```python
from build123d import *

# Parameters (mm, degrees)
F0_R     = 3
F1_DEPTH = 3.95
F0_R_2   = 2.499
F0_R_3   = 2.495
F2_DEPTH = 3.45
F3_R     = 3.69999


# Not quite as in the source:
# - a fillet or chamfer is up to 0.001 mm smaller than in the source, because OpenCascade refuses the exact size


with BuildPart() as f1:
    # F0 (on Front) → F1 (new body, symmetric)
    with BuildSketch(Plane.XZ):
        Polygon((15.7, -3.7), (15.7, 0), (15.7, 3.7), (-15.7, 3.7), (-15.7, -3.7), align=None)
        with BuildLine():
            ThreePointArc((-12.8998169675, 2.8618751589), (-11.9998409744, 2.9999999958), (-11.0998796299, 2.8617797468))
            Line((-11.0998796299, 2.8617797468), (-11.0998796299, 0.8996879915))
            Line((-11.0998796299, 0.8996879915), (-9.1380842923, 0.8996879915))
            ThreePointArc((-9.1380842923, 0.8996879915), (-9.0000000001, -2.51387e-05), (-9.1380993707, -0.8997359546))
            Line((-9.1380993707, -0.8997359546), (-11.0998796299, -0.8997359546))
            Line((-11.0998796299, -0.8997359546), (-11.0998796299, -2.8617797468))
            ThreePointArc((-11.0998796299, -2.8617797468), (-11.9998409744, -2.9999999958), (-12.8998169675, -2.8618751589))
            Line((-12.8998169675, -2.8618751589), (-12.8998169675, -0.8997359546))
            Line((-12.8998169675, -0.8997359546), (-14.8619006293, -0.8997359546))
            ThreePointArc((-14.8619006293, -0.8997359546), (-14.9999999999, -2.51387e-05), (-14.8619157077, 0.8996879915))
            Line((-14.8619157077, 0.8996879915), (-12.8998169675, 0.8996879915))
            Line((-12.8998169675, 0.8996879915), (-12.8998169675, 2.8618751589))
        make_face(mode=Mode.SUBTRACT)
        with Locations((-4, 0)):
            Circle(F0_R, mode=Mode.SUBTRACT)
        with Locations((4, 0)):
            Circle(F0_R, mode=Mode.SUBTRACT)
        with Locations((12, 0)):
            Circle(F0_R, mode=Mode.SUBTRACT)
    extrude(amount=F1_DEPTH, both=True)

    # F0 (on Front) → F2 (join, symmetric)
    with BuildSketch(Plane.XZ):
        with Locations((-4, 0)):
            Circle(F0_R)
        with Locations((-4, 0)):
            Circle(F0_R_2, mode=Mode.SUBTRACT)
        with Locations((4, 0)):
            Circle(F0_R)
        with Locations((4, 0)):
            Circle(F0_R_3, mode=Mode.SUBTRACT)
        with Locations((12, 0)):
            Circle(F0_R)
        with Locations((12, 0)):
            Circle(F0_R_2, mode=Mode.SUBTRACT)
    extrude(amount=F2_DEPTH, both=True)

    # F3 (radius 3.7 in the source; OpenCascade refuses exactly that, so slightly less here)
    f3_edges = [f1.edges().sort_by_distance(p)[0] for p in [
        (-15.7, 0, 3.7),
        (-15.7, 0, -3.7),
        (15.7, 0, 3.7),
        (15.7, 0, -3.7),
    ]]
    fillet(f3_edges, radius=F3_R)


solid = f1.part
```
Part model, mm, in its own coordinate system. A direction names the side the tool comes from. Round coordinates to 2 decimals unless told otherwise and drop trailing zeros. Write each loop counter-clockwise with the first axis right and the second up, starting at its lowest first coordinate (ties: lowest second). Pieces come first, ordered by that corner, then holes.
Item 1: Probe L1, parallel to Z at x = 4, y = -3.7; L2, parallel to Z at x = 12, y = -1.25; L3, parallel to X at y = 0.5, z = 2.25. List the from-to ranges inside material, lowest first.
Results:
L1: z = -3.7 to -3, 3 to 3.7
L2: z = -3.7 to -2.5, 2.5 to 3.7
L3: x = -14.94 to -12.9, -11.1 to -5.09, -2.91 to 2.92, 5.08 to 10.91, 13.09 to 14.94
Item 2: Cut at A-A, the plane x = 4. Give the cut face in (y, z) (3 decimals).
Results:
outline: (-3.95, -3.7) - (3.95, -3.7) - (3.95, -3) - (3.45, -3) - (3.45, -2.495) - (-3.45, -2.495) - (-3.45, -3) - (-3.95, -3) - close; (-3.95, 3) - (-3.45, 3) - (-3.45, 2.495) - (3.45, 2.495) - (3.45, 3) - (3.95, 3) - (3.95, 3.7) - (-3.95, 3.7) - close
Item 3: Drop flat-ended pins along their axis: pin 1 Ø1 at (y, z) = (0, -1.5) entering from +X; pin 2 Ø3.5 at (x, z) = (12, 0) entering from +Y; pin 3 Ø2 at (x, y) = (-14, 2) entering from -Z; pin 4 Ø1 at (y, z) = (-0.5, 1.5) entering from -X. Give the stop position or say it passes through.
Results:
pin 1: stops at x = 15.56
pin 2: passes through
pin 3: stops at z = -3.56
pin 4: stops at x = -15.56
Item 4: Cut at C-C, the plane x = -4. Give the cut face in (y, z), plus the area to 3 significant figures.
Results:
outline: (-3.95, -3.7) - (3.95, -3.7) - (3.95, -3) - (3.45, -3) - (3.45, -2.5) - (-3.45, -2.5) - (-3.45, -3) - (-3.95, -3) - close; (-3.95, 3) - (-3.45, 3) - (-3.45, 2.5) - (3.45, 2.5) - (3.45, 3) - (3.95, 3) - (3.95, 3.7) - (-3.95, 3.7) - close
area: 18.0 mm2
Item 5: Which spindle directions (+Z, -Z, +X, -X, +Y, -Y) get a long thin tool onto all of the face, cutting with end or side? Do faces 1 (the cylindrical face through (14.64, 0.06, -2.59)), 2 (the cylindrical face through (-14.59, 0.06, -2.64)), 3 (the flat face through (2, -3.45, 2)), 4 (the flat face through (-10, 0, 0.9)), 5 (the flat face through (-6, 3.45, 2)). Say none if no direction does.
Results:
face 1: -Z, +X, +Y, -Y
face 2: -Z, -X, +Y, -Y
face 3: -Y
face 4: +Y, -Y
face 5: +Y
Item 6: Two-plate mould, pull along Z, no slides. Class faces 6 (the cylindrical face through (-1.14, 3.7, 0.9)), 7 (the flat face through (0, 0, -3.7)), 8 (the flat face through (0, 0, 3.7)): +Z half, -Z half, draft (parallel to the pull), parting line (faces both ways), or undercut.
Results:
face 6: undercut
face 7: -Z half
face 8: +Z half
Item 7: Cut at B-B, the plane y = -0.75. Count the separate pieces of the cut face and the enclosed holes in it, plus the area to 3 significant figures.
Results:
separate pieces: 1
enclosed holes: 4
area: 144 mm2
